Can you work these out from the model? Positions are in its coordinate system, mm. Coordinates: 2 decimals unless noted, no trailing zeros. Loops run counter-clockwise (first coordinate to the right, second up) from the corner with the lowest first, then second, coordinate; pieces in that order, holes last. Notation, with made-up numbers: M 24,-34 L 28,-34 A7 cw 28,-23 Z; hole C 83.5,84 d7. An arc over 180 degrees is marked long. Answer as a JSON object with one key per item and string values. Group by question number.
Item 1: We'd pull the mould along Z, two halves only. Please class faces 1 (the cylindrical face through (17.86, 1.25, -24.16)), 2 (the flat face through (1, 2.54, -1)), 3 (the cylindrical face through (-39.08, 1.25, -25.54)), 4 (the flat face through (74.02, 1.25, -21.31)): +Z half, -Z half, draft (parallel to the pull), parting line (faces both ways), or undercut.
Item 2: Suppose I cut it at C-C (z = 36.5). Write out the boundary of the cut face in (x, y).
Item 3: Suppose I cut it at B-B (y = 1.6). Count the separate pieces of the cut face and the enclosed holes in it, then the cut area to 3 significant figures.
Item 4: If I drill on line 1 (Z direction, x = -56.5, y = 1.35) (1 decimal); line 2 (X direction, y = 0.35, z = -1.5); line 3 (X direction, y = 0.8, z = -11), over which ranges is the centre line in solid material (lowest first)?
Item 5: Suppose I cut it at A-A (x = -60.5). Write out the boundary of the cut face in (y, z) (1 decimal), then the cut area to 3 significant figures.
Item 6: I'm going to push flat-ended pins straight in: pin 1 Ø0.8 at (x, y) = (34, 1.5) entering from +Z; pin 2 Ø1.5 at (y, z) = (1, -30.5) entering from -X. Where does each tip first touch, or does it pass through?
```python
from build123d import *

# Parameters (mm, degrees)
BOSS_EXTRUDE1_DEPTH = 2.54
SKETCH3_W           = 28
SKETCH3_H           = 11
SKETCH3_W_2         = 10
SKETCH3_H_2         = 28
CUT_EXTRUDE_1_DEPTH = 10
CUT_EXTRUDE2_DEPTH  = 2.54
SKETCH_1_W          = 45
SKETCH_1_H          = 3.5
CUT_EXTRUDE_2_DEPTH = 2.54
FILLET_1_R          = 1
SKETCH_2_R          = 1.35
SKETCH_2_R_2        = 1.3
CUT_EXTRUDE_5_DEPTH = 2.54


with BuildPart() as part:
    # Sketch1 → Boss-Extrude1 (new body)
    with BuildSketch(Plane(origin=(0, 0, 0), x_dir=(1, 0, 0), z_dir=(0, 1, 0))):
        with BuildLine():
            Line((-23.244816627, 44.45), (23.244816627, 44.45))
            ThreePointArc((23.244816627, 44.45), (24.583514169, 44.270437622), (25.827574029, 43.744444444))
            ThreePointArc((25.827574029, 43.744444444), (35.740062311, 36.101079569), (43.482663438, 26.265909091))
            ThreePointArc((43.482663438, 26.265909091), (45.334600658, 24.468164919), (47.830929781, 23.8125))
            Line((47.830929781, 23.8125), (71.516875, 23.8125))
            Line((71.516875, 23.8125), (76.596875, 18.7325))
            Line((76.596875, 18.7325), (76.596875, -18.7325))
            Line((76.596875, -18.7325), (71.516875, -23.8125))
            Line((71.516875, -23.8125), (47.830929781, -23.8125))
            ThreePointArc((47.830929781, -23.8125), (45.334600658, -24.468164919), (43.482663438, -26.265909091))
            ThreePointArc((43.482663438, -26.265909091), (35.740062311, -36.101079569), (25.827574029, -43.744444444))
            ThreePointArc((25.827574029, -43.744444444), (24.583514169, -44.270437622), (23.244816627, -44.45))
            Line((23.244816627, -44.45), (-23.244816627, -44.45))
            ThreePointArc((-23.244816627, -44.45), (-24.583514169, -44.270437622), (-25.827574029, -43.744444444))
            ThreePointArc((-25.827574029, -43.744444444), (-35.740062311, -36.101079569), (-43.482663438, -26.265909091))
            ThreePointArc((-43.482663438, -26.265909091), (-45.334600658, -24.468164919), (-47.830929781, -23.8125))
            Line((-47.830929781, -23.8125), (-71.516875, -23.8125))
            Line((-71.516875, -23.8125), (-76.596875, -18.7325))
            Line((-76.596875, -18.7325), (-76.596875, 18.7325))
            Line((-76.596875, 18.7325), (-71.516875, 23.8125))
            Line((-71.516875, 23.8125), (-47.830929781, 23.8125))
            ThreePointArc((-47.830929781, 23.8125), (-45.334600658, 24.468164919), (-43.482663438, 26.265909091))
            ThreePointArc((-43.482663438, 26.265909091), (-35.740062311, 36.101079569), (-25.827574029, 43.744444444))
            ThreePointArc((-25.827574029, 43.744444444), (-24.583514169, 44.270437622), (-23.244816627, 44.45))
        make_face()
    extrude(amount=BOSS_EXTRUDE1_DEPTH)

    # Sketch3 → 切除-拉伸1 (cut)
    with BuildSketch(Plane(origin=(0, 2.54, 0), x_dir=(1, 0, 0), z_dir=(0, 1, 0))):
        with Locations((0, 28)):
            Rectangle(SKETCH3_W, SKETCH3_H)
        with Locations((0, -28)):
            Rectangle(SKETCH3_W, SKETCH3_H)
        with Locations((-33, 0)):
            Rectangle(SKETCH3_W_2, SKETCH3_H_2)
        with Locations((33, 0)):
            Rectangle(SKETCH3_W_2, SKETCH3_H_2)
    extrude(amount=-CUT_EXTRUDE_1_DEPTH, mode=Mode.SUBTRACT)

    # Sketch4 → Cut-Extrude2 (cut)
    with BuildSketch(Plane(origin=(0, 2.54, 0), x_dir=(1, 0, 0), z_dir=(0, 1, 0))):
        with BuildLine():
            Line((44.592875, 14.605), (67.452875, 14.605))
            ThreePointArc((67.452875, 14.605), (68.350900612, 14.233025612), (68.722875, 13.335))
            Line((68.722875, 13.335), (68.722875, 12.065))
            ThreePointArc((68.722875, 12.065), (68.350900612, 11.166974388), (67.452875, 10.795))
            Line((67.452875, 10.795), (44.592875, 10.795))
            ThreePointArc((44.592875, 10.795), (43.694849388, 11.166974388), (43.322875, 12.065))
            Line((43.322875, 12.065), (43.322875, 13.335))
            ThreePointArc((43.322875, 13.335), (43.694849388, 14.233025612), (44.592875, 14.605))
        make_face()
        with BuildLine():
            Line((68.722875, -13.335), (68.722875, -12.065))
            ThreePointArc((68.722875, -12.065), (68.350900612, -11.166974388), (67.452875, -10.795))
            Line((67.452875, -10.795), (44.592875, -10.795))
            ThreePointArc((44.592875, -10.795), (43.694849388, -11.166974388), (43.322875, -12.065))
            Line((43.322875, -12.065), (43.322875, -13.335))
            ThreePointArc((43.322875, -13.335), (43.694849388, -14.233025612), (44.592875, -14.605))
            Line((44.592875, -14.605), (67.452875, -14.605))
            ThreePointArc((67.452875, -14.605), (68.350900612, -14.233025612), (68.722875, -13.335))
        make_face()
        with BuildLine():
            Line((-44.592875, -14.605), (-67.452875, -14.605))
            ThreePointArc((-67.452875, -14.605), (-68.350900612, -14.233025612), (-68.722875, -13.335))
            Line((-68.722875, -13.335), (-68.722875, -12.065))
            ThreePointArc((-68.722875, -12.065), (-68.350900612, -11.166974388), (-67.452875, -10.795))
            Line((-67.452875, -10.795), (-44.592875, -10.795))
            ThreePointArc((-44.592875, -10.795), (-43.694849388, -11.166974388), (-43.322875, -12.065))
            Line((-43.322875, -12.065), (-43.322875, -13.335))
            ThreePointArc((-43.322875, -13.335), (-43.694849388, -14.233025612), (-44.592875, -14.605))
        make_face()
        with BuildLine():
            Line((-68.722875, 13.335), (-68.722875, 12.065))
            ThreePointArc((-68.722875, 12.065), (-68.350900612, 11.166974388), (-67.452875, 10.795))
            Line((-67.452875, 10.795), (-44.592875, 10.795))
            ThreePointArc((-44.592875, 10.795), (-43.694849388, 11.166974388), (-43.322875, 12.065))
            Line((-43.322875, 12.065), (-43.322875, 13.335))
            ThreePointArc((-43.322875, 13.335), (-43.694849388, 14.233025612), (-44.592875, 14.605))
            Line((-44.592875, 14.605), (-67.452875, 14.605))
            ThreePointArc((-67.452875, 14.605), (-68.350900612, 14.233025612), (-68.722875, 13.335))
        make_face()
    extrude(amount=-CUT_EXTRUDE2_DEPTH, mode=Mode.SUBTRACT)

    # 草图1 → 切除-拉伸2 (cut)
    with BuildSketch(Plane(origin=(0, 2.54, 0), x_dir=(1, 0, 0), z_dir=(0, 1, 0))):
        with Locations((0, 5.75)):
            Rectangle(SKETCH_1_W, SKETCH_1_H)
        with Locations((0, 15.75)):
            Rectangle(SKETCH_1_W, SKETCH_1_H)
        with Locations((0, -5.75)):
            Rectangle(SKETCH_1_W, SKETCH_1_H)
        with Locations((0, -15.75)):
            Rectangle(SKETCH_1_W, SKETCH_1_H)
    extrude(amount=-CUT_EXTRUDE_2_DEPTH, mode=Mode.SUBTRACT)

    # 圆角1
    fillet_1_edges = [part.edges().sort_by_distance(p)[0] for p in [
        (-28, 1.27, -14),
        (-28, 1.27, 14),
        (-38, 1.27, 14),
        (-38, 1.27, -14),
        (38, 1.27, 14),
        (28, 1.27, 14),
        (28, 1.27, -14),
        (38, 1.27, -14),
        (22.5, 1.27, 17.5),
        (22.5, 1.27, 14),
        (-22.5, 1.27, 14),
        (-22.5, 1.27, 17.5),
        (22.5, 1.27, -17.5),
        (-22.5, 1.27, -17.5),
        (-22.5, 1.27, -14),
        (22.5, 1.27, -14),
        (22.5, 1.27, 7.5),
        (22.5, 1.27, 4),
        (-22.5, 1.27, 4),
        (-22.5, 1.27, 7.5),
        (-22.5, 1.27, -7.5),
        (-22.5, 1.27, -4),
        (22.5, 1.27, -4),
        (22.5, 1.27, -7.5),
        (14, 1.27, -33.5),
        (14, 1.27, -22.5),
        (-14, 1.27, -22.5),
        (-14, 1.27, -33.5),
        (14, 1.27, 33.5),
        (-14, 1.27, 33.5),
        (-14, 1.27, 22.5),
        (14, 1.27, 22.5),
    ]]
    fillet(fillet_1_edges, radius=FILLET_1_R)

    # 草图2 → 切除-拉伸5 (cut)
    with BuildSketch(Plane.XZ):
        with Locations((19.207738721, -24.223015039)):
            Circle(SKETCH_2_R)
        with Locations((19.207738721, 24.776984961)):
            Circle(SKETCH_2_R)
        with Locations((-38.792261279, -24.223015039)):
            Circle(SKETCH_2_R)
        with Locations((-38.792261279, 24.776984961)):
            Circle(SKETCH_2_R_2)
    extrude(amount=-CUT_EXTRUDE_5_DEPTH, mode=Mode.SUBTRACT)


solid = part.part
```
From the geometry:
{
 "1": {"face 1": "undercut", "face 2": "draft", "face 3": "undercut", "face 4": "-Z half"},
 "2": {"outline": "M -35.33,0 L 35.33,0 L 35.33,2.54 L -35.33,2.54 Z"},
 "3": {"separate pieces": "1", "enclosed holes": "16", "area": "8,080 mm2"},
 "4": {"line 1": "-23.8 to -14.6, -10.8 to 10.8, 14.6 to 23.8", "line 2": "-76.6 to -38, -28 to 28, 38 to 76.6", "line 3": "-76.6 to -68.14, -43.9 to -38, -28 to 28, 38 to 43.9, 68.14 to 76.6"},
 "5": {"outline": "M 0,-23.8 L 2.5,-23.8 L 2.5,-14.6 L 0,-14.6 Z; M 0,-10.8 L 2.5,-10.8 L 2.5,10.8 L 0,10.8 Z; M 0,14.6 L 2.5,14.6 L 2.5,23.8 L 0,23.8 Z", "area": "102 mm2"},
 "6": {"pin 1": "z = 38.1", "pin 2": "x = -41.18"}
}
